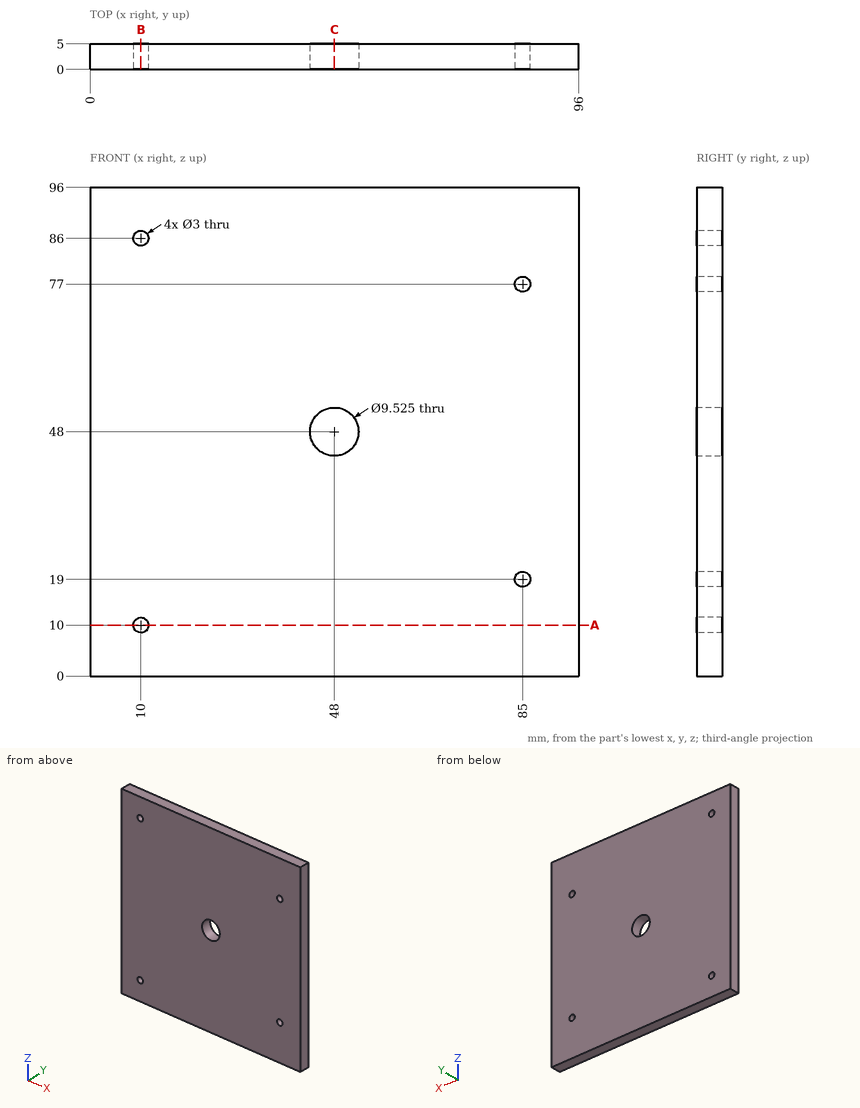
Can you work these out from the drawing? Everything is in mm from the part's minimum corner. Round coordinates to 2 decimals unless told otherwise and drop trailing zeros. Write each loop counter-clockwise with the first axis right and the second up, starting at its lowest first coordinate (ties: lowest second). Pieces come first, ordered by that corner, then holes. Notation, with made-up numbers: (-33, -11.75) - (-1, -11.75) arc R18 ccw to (-1, 14.25) - close; hole circle Ø9 at (-12, -25.5). An arc over 180 degrees is marked (long way). Write each question's results on one line, items separated by ' | '. Start each with the question number.
1) For pin 1 Ø5.5 at (x, z) = (48, 48) entering from +Y, with a flat end and sliding along its axis, tell me the tip position at first contact or that it passes through.
2) Suppose I cut it at C-C (x = 48). List the corners of the cut face in (y, z) for me, and give its area (3 significant figures).
3) Suppose I cut it at A-A (z = 10). List the corners of the cut face in (x, y) for me.
4) Suppose I cut it at B-B (x = 10). List the corners of the cut face in (y, z) for me, and give its area (3 significant figures).
5) Please list where these lines run through material, in increasing order: line 1 (Z direction, x = 10, y = 1.6); line 2 (Z direction, x = 48, y = 3.25); line 3 (Z direction, x = 85, y = 2.45).
Here are the results:
1) pin 1: passes through
2) outline: (0, 0) - (5, 0) - (5, 43.24) - (0, 43.24) - close; (0, 52.76) - (5, 52.76) - (5, 96) - (0, 96) - close | area: 432 mm2
3) outline: (0, 0) - (8.5, 0) - (8.5, 5) - (0, 5) - close; (11.5, 0) - (96, 0) - (96, 5) - (11.5, 5) - close
4) outline: (0, 0) - (5, 0) - (5, 8.5) - (0, 8.5) - close; (0, 11.5) - (5, 11.5) - (5, 84.5) - (0, 84.5) - close; (0, 87.5) - (5, 87.5) - (5, 96) - (0, 96) - close | area: 450 mm2
5) line 1: z = 0 to 8.5, 11.5 to 84.5, 87.5 to 96 | line 2: z = 0 to 43.24, 52.76 to 96 | line 3: z = 0 to 17.5, 20.5 to 75.5, 78.5 to 96
